from build123d import *

# Parameters (mm, degrees)
ESQUISSE2_R                  = 2
ENL_V_MAT_EXTRU_1_DEPTH      = 97.788429061
CHANFREIN1_SIZE              = 1
NERVURE11_REACH              = 101.403
ESQUISSE5_WALL_W             = 253.94775955
ESQUISSE5_WALL_H             = 3
R_P_TITION_CIRCULAIRE1_COUNT = 6


with BuildPart() as part:
    # Esquisse1 → Révolution1 (revolve)
    with BuildSketch(Plane.XY):
        Polygon((-8, 0), (-34, 0), (-34, 3), (-19, 3), (-14, 3), (-14, 8), (-14, 87), (-11, 87), (-11, 80), (-8, 80), align=None)
    revolve(axis=Axis((0, 5.729166667, 0), (0, -1, 0)))

    # Esquisse2 → Enlèv. mat.-Extru.1 (cut, through all)
    with BuildSketch(Plane(origin=(0, 3, 0), x_dir=(1, 0, 0), z_dir=(0, 1, 0))):
        with Locations(Location((0, 30, 0), (0, 0, 180))):
            Circle(ESQUISSE2_R)
        with Locations(Location((25.980762114, 15, 0), (0, 0, 180))):
            Circle(ESQUISSE2_R)
        with Locations(Location((25.980762114, -15, 0), (0, 0, 180))):
            Circle(ESQUISSE2_R)
        with Locations(Location((0, -30, 0), (0, 0, 180))):
            Circle(ESQUISSE2_R)
        with Locations(Location((-25.980762114, -15, 0), (0, 0, 180))):
            Circle(ESQUISSE2_R)
        with Locations(Location((-25.980762114, 15, 0), (0, 0, 180))):
            Circle(ESQUISSE2_R)
    extrude(amount=-ENL_V_MAT_EXTRU_1_DEPTH, mode=Mode.SUBTRACT)

    # Chanfrein1
    chanfrein1_edges = [part.edges().sort_by_distance(p)[0] for p in [
        (11, 87, 0),
    ]]
    chamfer(chanfrein1_edges, length=CHANFREIN1_SIZE)

    # Esquisse5 wall → Nervure11 (add, up to next)
    with BuildSketch(Plane(origin=(23, 28, 0), x_dir=(0.338719468273, -0.940887411869, 0), z_dir=(0.940887411869, 0.338719468273, 0)), mode=Mode.PRIVATE) as nervure11_sk1:
        Rectangle(ESQUISSE5_WALL_W, ESQUISSE5_WALL_H)
    nervure11_tool1 = extrude(nervure11_sk1.sketch, amount=-NERVURE11_REACH, mode=Mode.PRIVATE) - part.part
    nervure11 = nervure11_tool1.solids().sort_by_distance((23, 28, 0))[0]
    add(nervure11)

    # Répétition circulaire1: Nervure11 ×6 about axis
    r_p_tition_circulaire1_axis = Axis((0, 0, 0), (0, 1, 0))
    for i in range(1, R_P_TITION_CIRCULAIRE1_COUNT):
        add(nervure11.rotate(r_p_tition_circulaire1_axis, i * 360 / R_P_TITION_CIRCULAIRE1_COUNT))


solid = part.part
Source: CAD feature listing. Evaluate the final solid. Frame: model axes, mm. A direction names the side the tool comes from. Round coordinates to 2 decimals unless told otherwise and drop trailing zeros. Loops run counter-clockwise (first coordinate to the right, second up) from the corner with the lowest first, then second, coordinate; pieces in that order, holes last. Notation, with made-up numbers: (67.5, 12.5) - (95.5, 12.5) arc R32 cw to (95.5, 44.5) - close; hole circle Ø4 at (51.5, 84). An arc over 180 degrees is marked (long way). Write item = value, one per line. Start each with the question number.
(1) Pin query (flat end, axial travel): pin 1 (14.5 mm diameter, centred on x = -21.5, y = 37.5, fed in from +Z); pin 2 (1 mm diameter, centred on x = -1.5, y = 34.5, fed in from +Z); pin 3 (8 mm diameter, centred on x = -19, z = -10, fed in from +Y); pin 4 (10 mm diameter, centred on x = -1, z = 5, fed in from -Y). Return the tip coordinate at first contact, or that it passes through.
(2) Ray query, line 1 along Z through (x, y) = (0, 2.05); line 2 along Z through (x, y) = (-16.5, 5.5); line 3 along Z through (x, y) = (11.5, 11). Return the intervals inside material, ascending. Write a range as from..to.
(3) Pull-direction query (Z, two-part tool) for faces 4 (the face through (-26, 2, 17)), 5 (the face through (7, 0, 7)), 6 (the face through (3.03, 44.41, 13.67)), 7 (the face through (11.435, 28.463, 19.764)); classes: +Z half, -Z half, draft (parallel to the pull), parting line (faces both ways), or undercut.
(4) Section query C-C, the plane y = 30.5. Output: boundary loops of the cut face in (x, z).
(5) Section query D-D, the plane z = 0. Output: boundary loops of the cut face in (x, y).
(6) Section query B-B, the plane z = -30. Output: boundary loops of the cut face in (x, y), plus the area to 3 significant figures.
(7) Section query A-A, the plane x = 0. Output: boundary loops of the cut face in (y, z).
(8) Set-up query: faces 1 (the face through (-8.955, 21.323, -18.51)), 2 (the face through (11.553, 21.323, -17.01)), 3 (the face through (-8.955, 21.323, 18.51)). Return all of +Z, -Z, +X, -X, +Y, -Y with unobstructed straight access to the full face (end or side cutting, diameter ignored); none if empty.
Conclusion:
q1.pin_1 = 1.5
q1.pin_2 = 13.96
q1.pin_3 = 3
q1.pin_4 = 0
q2.line_1 = -34..-32, -28..-8, 8..28, 32..34
q2.line_2 = -26.38..-25.58, -1.5..1.5, 25.58..26.38
q2.line_3 = -22.92..-16.92, -7.98..7.98, 16.92..22.92
q3.face_4 = undercut
q3.face_5 = draft
q3.face_6 = undercut
q3.face_7 = +Z half
q4.outline = (-22.1, -1.5) - (-13.92, -1.5) arc R14 ccw to (-8.26, -11.3) - (-12.35, -18.39) - (-9.75, -19.89) - (-5.66, -12.8) arc R14 ccw to (5.66, -12.8) - (9.75, -19.89) - (12.35, -18.39) - (8.26, -11.3) arc R14 ccw to (13.92, -1.5) - (22.1, -1.5) - (22.1, 1.5) - (13.92, 1.5) arc R14 ccw to (8.26, 11.3) - (12.35, 18.39) - (9.75, 19.89) - (5.66, 12.8) arc R14 ccw to (-5.66, 12.8) - (-9.75, 19.89) - (-12.35, 18.39) - (-8.26, 11.3) arc R14 ccw to (-13.92, 1.5) - (-22.1, 1.5) - close; hole circle Ø16 at (0, 0)
q5.outline = (-34, 0) - (-8, 0) - (-8, 80) - (-11, 80) - (-11, 86) - (-12, 87) - (-14, 87) - (-14, 53) - (-32, 3) - (-34, 3) - close; (8, 0) - (34, 0) - (34, 3) - (32, 3) - (14, 53) - (14, 87) - (12, 87) - (11, 86) - (11, 80) - (8, 80) - close
q6.outline = (-16, 0) - (-2, 0) - (-2, 3) - (-16, 3) - close; (2, 0) - (16, 0) - (16, 3) - (2, 3) - close
q6.area = 84.0 mm2
q7.outline = (0, -34) - (3, -34) - (3, -32) - (0, -32) - close; (0, -28) - (3, -28) - (3, -14) - (87, -14) - (87, -12) - (86, -11) - (80, -11) - (80, -8) - (0, -8) - close; (0, 8) - (80, 8) - (80, 11) - (86, 11) - (87, 12) - (87, 14) - (3, 14) - (3, 28) - (0, 28) - close; (0, 32) - (3, 32) - (3, 34) - (0, 34) - close
q8.face_1 = -Z, +Y
q8.face_2 = +X, +Y
q8.face_3 = +Z, +Y
